Here's how the part is built. I have some questions about the finished solid (model axes, mm). A direction names the side the tool comes from. Round coordinates to 2 decimals unless told otherwise and drop trailing zeros. Loops run counter-clockwise (first coordinate to the right, second up) from the corner with the lowest first, then second, coordinate; pieces in that order, holes last. Notation, with made-up numbers: M 84.25,32.5 L 120.25,32.5 A20 ccw 120.25,53.5 Z; hole C 3.25,43 d7. An arc over 180 degrees is marked long. Use a Markdown table: item, result.
from build123d import *

# Parameters (mm, degrees)
SKETCH1_R                                    = 40
SKETCH1_R_2                                  = 20
BOSS_EXTRUDE1_DEPTH                          = 8.5
SKETCH2_R                                    = 1
CUT_EXTRUDE2_DEPTH                           = 58.203583804
SKETCH2_6_R                                  = 3
SKETCH2_6_R_2                                = 1
BOSS_EXTRUDE3_DEPTH                          = 8.5
CIRPATTERN1_COUNT                            = 4
CUT_EXTRUDE4_DEPTH                           = 62.402361518
CIRPATTERN3_COUNT                            = 4
SKETCH7_R                                    = 21
CUT_EXTRUDE5_DEPTH                           = 7
SKETCH8_R                                    = 1
OUTER_RETAINER_M2_TAPPED_ENVELOPE_DEPTH      = 4.3
SKETCH9_R                                    = 1
REVB_OLDHAM_FOUR_M2_BLIND_THREAD_MAJOR_DEPTH = 5.8
SKETCH10_R                                   = 1.51
REVB_OLDHAM_FOUR_D3P02_PILOT_POCKETS_DEPTH   = 1.1


with BuildPart() as part:
    # Sketch1 → Boss-Extrude1 (new body)
    with BuildSketch(Plane(origin=(0, 0, 0), x_dir=(1, 0, 0), z_dir=(0, 1, 0))):
        with Locations(Location((0, 0, 0), (0, 0, 270))):
            Circle(SKETCH1_R)
        with Locations(Location((0, 0, 0), (0, 0, 270))):
            Circle(SKETCH1_R_2, mode=Mode.SUBTRACT)
    extrude(amount=BOSS_EXTRUDE1_DEPTH)

    # Sketch2 → Cut-Extrude2 (cut, through all)
    with BuildSketch(Plane(origin=(0, 8.5, 0), x_dir=(1, 0, 0), z_dir=(0, 1, 0))):
        with Locations((40, 0)):
            Circle(SKETCH2_R)
    cut_extrude2 = extrude(amount=-CUT_EXTRUDE2_DEPTH, mode=Mode.SUBTRACT)

    # Sketch2_6 → Boss-Extrude3 (add)
    with BuildSketch(Plane(origin=(0, 8.5, 0), x_dir=(1, 0, 0), z_dir=(0, 1, 0))):
        with Locations((40, 0)):
            Circle(SKETCH2_6_R)
        with Locations(Location((40, 0, 0), (0, 0, 270))):
            Circle(SKETCH2_6_R_2, mode=Mode.SUBTRACT)
    boss_extrude3 = extrude(amount=-BOSS_EXTRUDE3_DEPTH)

    # CirPattern1: Cut-Extrude2, Boss-Extrude3 ×4 about axis
    cirpattern1_axis = Axis((0, 0, 0), (0, 1, 0))
    add([cut_extrude2.rotate(cirpattern1_axis, i * 360 / CIRPATTERN1_COUNT) for i in range(1, CIRPATTERN1_COUNT)], mode=Mode.SUBTRACT)
    add([boss_extrude3.rotate(cirpattern1_axis, i * 360 / CIRPATTERN1_COUNT) for i in range(1, CIRPATTERN1_COUNT)])

    # Sketch4 → Cut-Extrude4 (cut, through all)
    with BuildSketch(Plane(origin=(0, 8.5, 0), x_dir=(1, 0, 0), z_dir=(0, 1, 0))):
        with BuildLine():
            Line((-27.170578067, -25.049257724), (-17.377149148, -15.255828804))
            ThreePointArc((-17.377149148, -15.255828804), (-15.255828804, -15.255828804), (-15.255828804, -17.377149148))
            Line((-15.255828804, -17.377149148), (-25.049257724, -27.170578067))
            ThreePointArc((-25.049257724, -27.170578067), (-27.170578067, -27.170578067), (-27.170578067, -25.049257724))
        make_face()
    cut_extrude4 = extrude(amount=-CUT_EXTRUDE4_DEPTH, mode=Mode.SUBTRACT)

    # CirPattern3: Cut-Extrude4 ×4 about axis
    cirpattern3_axis = Axis((0, 0, 0), (0, 1, 0))
    for i in range(1, CIRPATTERN3_COUNT):
        add(cut_extrude4.rotate(cirpattern3_axis, i * 360 / CIRPATTERN3_COUNT), mode=Mode.SUBTRACT)

    # Sketch7 → Cut-Extrude5 (cut)
    with BuildSketch(Plane(origin=(0, 8.5, 0), x_dir=(1, 0, 0), z_dir=(0, 1, 0))):
        with Locations(Location((0, 0, 0), (0, 0, 270))):
            Circle(SKETCH7_R)
    extrude(amount=-CUT_EXTRUDE5_DEPTH, mode=Mode.SUBTRACT)

    # Sketch8 → Outer_Retainer_M2_Tapped_Envelope (cut)
    with BuildSketch(Plane(origin=(0, 8.5, 0), x_dir=(1, 0, 0), z_dir=(0, 1, 0))):
        with Locations(Location((0.720053396, -22.48847534, 0), (0, 0, 270))):
            Circle(SKETCH8_R)
        with Locations(Location((19.115564239, 11.867822203, 0), (0, 0, 270))):
            Circle(SKETCH8_R)
        with Locations(Location((-19.835617634, 10.620653137, 0), (0, 0, 270))):
            Circle(SKETCH8_R)
    extrude(amount=-OUTER_RETAINER_M2_TAPPED_ENVELOPE_DEPTH, mode=Mode.SUBTRACT)

    # Sketch9 → RevB_Oldham_Four_M2_Blind_Thread_Major (cut)
    with BuildSketch(Plane.XZ):
        with Locations(Location((27.716385975, 11.480502971, 0), (0, 0, 270))):
            Circle(SKETCH9_R)
        with Locations(Location((-11.480502971, 27.716385975, 0), (0, 0, 270))):
            Circle(SKETCH9_R)
        with Locations(Location((-27.716385975, -11.480502971, 0), (0, 0, 270))):
            Circle(SKETCH9_R)
        with Locations(Location((11.480502971, -27.716385975, 0), (0, 0, 270))):
            Circle(SKETCH9_R)
    extrude(amount=-REVB_OLDHAM_FOUR_M2_BLIND_THREAD_MAJOR_DEPTH, mode=Mode.SUBTRACT)

    # Sketch10 → RevB_Oldham_Four_D3p02_Pilot_Pockets (cut)
    with BuildSketch(Plane.XZ):
        with Locations(Location((27.716385975, 11.480502971, 0), (0, 0, 270))):
            Circle(SKETCH10_R)
        with Locations(Location((-11.480502971, 27.716385975, 0), (0, 0, 270))):
            Circle(SKETCH10_R)
        with Locations(Location((-27.716385975, -11.480502971, 0), (0, 0, 270))):
            Circle(SKETCH10_R)
        with Locations(Location((11.480502971, -27.716385975, 0), (0, 0, 270))):
            Circle(SKETCH10_R)
    extrude(amount=-REVB_OLDHAM_FOUR_D3P02_PILOT_POCKETS_DEPTH, mode=Mode.SUBTRACT)


solid = part.part
1. For pin 1 Ø1.5 at (y, z) = (2, -8.5) entering from +X; pin 2 Ø2 at (x, z) = (27.5, 12) entering from -Y; pin 3 Ø1.5 at (x, z) = (11, -27.5) entering from -Y; pin 4 Ø1.5 at (y, z) = (4, -23.5) entering from -X, each with a flat end and sliding along its axis, tell me the tip position at first contact or that it passes through.
Answer sheet:
| item | result |
|---|---|
| pin 1 | x = 39.24 |
| pin 2 | y = 0 |
| pin 3 | y = 1.1 |
| pin 4 | x = -32.9 |
2. I need wall thicknesses on probe 1 along X at (y, z) = (6.5, 0); probe 2 along Z at (x, y) = (-12, 5.5); probe 3 along Z at (x, y) = (-40, 5.5). Which ranges of each line are inside material? Lowest first, please. Write a range as from..to.
Answer sheet:
| item | result |
|---|---|
| probe 1 | -43..-41, -39..-21, 21..39, 41..43 |
| probe 2 | -38.16..-17.23, 17.23..26.86, 28.57..38.16 |
| probe 3 | -3..-1, 1..3 |
3. Imagine slicing it at A-A, the plane z = 0. Write out the boundary of the cut face in (x, y), then the cut area to 3 significant figures.
Answer sheet:
| item | result |
|---|---|
| outline | M -43,0 L -41,0 L -41,8.5 L -43,8.5 Z; M -39,0 L -20,0 L -20,1.5 L -21,1.5 L -21,8.5 L -39,8.5 Z; M 20,0 L 39,0 L 39,8.5 L 21,8.5 L 21,1.5 L 20,1.5 Z; M 41,0 L 43,0 L 43,8.5 L 41,8.5 Z |
| area | 343 mm2 |
4. Imagine slicing it at B-B, the plane x = -6.5. Write out the boundary of the cut face in (y, z).
Answer sheet:
| item | result |
|---|---|
| outline | M 0,-39.47 L 8.5,-39.47 L 8.5,-19.97 L 1.5,-19.97 L 1.5,-18.91 L 0,-18.91 Z; M 0,18.91 L 1.5,18.91 L 1.5,19.97 L 8.5,19.97 L 8.5,39.47 L 0,39.47 Z |
5. Imagine slicing it at C-C, the plane x = 31.5. Write out the boundary of the cut face in (y, z).
Answer sheet:
| item | result |
|---|---|
| outline | M 0,-24.65 L 8.5,-24.65 L 8.5,24.65 L 0,24.65 Z |
6. We'd pull the mould along Z, two halves only. Please class faces 1 (the face through (28.002, 4.19, 28.564)), 2 (the face through (-10, 8.5, -19)), 3 (the face through (-19.535, 6.38, -9.667)): +Z half, -Z half, draft (parallel to the pull), parting line (faces both ways), or undercut.
Answer sheet:
| item | result |
|---|---|
| face 1 | +Z half |
| face 2 | draft |
| face 3 | undercut |
7. Which directions (+Z, -Z, +X, -X, +Y, -Y) give clear straight access to the entire face, cutting with the end or side of a thin tool? Please do faces 4 (the face through (19.416, 6.38, -10.914)), 5 (the face through (-22.34, 4.31, 20.22)), 6 (the face through (28.708, 3.417, 11.611)).
Answer sheet:
| item | result |
|---|---|
| face 4 | +Y |
| face 5 | +Y, -Y |
| face 6 | -Y |
